from build123d import *

# Parameters (mm, degrees)
SKETCH1_R           = 13.5
BOSS_EXTRUDE1_DEPTH = 5
SKETCH2_R           = 10.65
BOSS_EXTRUDE2_DEPTH = 9.9
SKETCH5_R           = 6.1
CUT_EXTRUDE1_DEPTH  = 10


with BuildPart() as part:
    # Sketch1 → Boss-Extrude1 (new body)
    with BuildSketch(Plane.XY):
        Circle(SKETCH1_R)
    extrude(amount=BOSS_EXTRUDE1_DEPTH)

    # Sketch2 → Boss-Extrude2 (add)
    with BuildSketch(Plane.XY.offset(5)):
        with Locations(Location((0, 0, 0), (0, 0, 180))):
            Circle(SKETCH2_R)
    extrude(amount=BOSS_EXTRUDE2_DEPTH)

    # Sketch5 → Cut-Extrude1 (cut)
    with BuildSketch(Plane.XY.offset(5)):
        Circle(SKETCH5_R)
    extrude(amount=CUT_EXTRUDE1_DEPTH, mode=Mode.SUBTRACT)


solid = part.part
For this review, take the finished solid that the model builds, in its own axes (mm). A direction names the side the tool comes from. Round coordinates to 2 decimals unless told otherwise and drop trailing zeros. Loops run counter-clockwise (first coordinate to the right, second up) from the corner with the lowest first, then second, coordinate; pieces in that order, holes last. Notation, with made-up numbers: (81.5, 8.5) - (134.5, 8.5) arc R12 cw to (134.5, 29.5) - close; hole circle Ø10 at (89, 17). An arc over 180 degrees is marked (long way). Use one line per item in the form item = value.
Item 1: Tool access review of faces 5 (the flat face through (-5, 5, 14.9)), 6 (the cylindrical face through (-10.158, -3.199, 9.881)): name each direction out of +Z, -Z, +X, -X, +Y, -Y from which nothing blocks a thin tool from reaching the whole face with its end or side.
Answers:
face_5 = +Z, +X, -X, +Y, -Y
face_6 = +Z
Item 2: Consider section D-D on z = 2.75. Write out the cut boundary in (x, y), then the cut area to 3 significant figures.
Answers:
outline = circle Ø27 at (0, 0)
area = 573 mm^2
Item 3: Mouldability with a two-part tool opening along Y and no side actions: class faces 1 (the cylindrical face through (-2.93, -13.18, 2.46)), 2 (the cylindrical face through (-6.094, 0.268, 9.881)), 3 (the flat face through (0, 0, 5)), 4 (the flat face through (-10.1, -3.9, 5)) as +Y half, -Y half, draft (parallel to the pull), parting line (faces both ways), or undercut.
Answers:
face_1 = parting line
face_2 = undercut
face_3 = undercut
face_4 = draft
Item 4: Consider section A-A on z = 8. Write out the cut boundary in (x, y).
Answers:
outline = circle Ø21.3 at (0, 0); hole circle Ø12.2 at (0, 0)
Item 5: Consider section B-B on x = 0. Write out the cut boundary in (y, z), then the cut area to 3 significant figures.
Answers:
outline = (-13.5, 0) - (13.5, 0) - (13.5, 5) - (10.65, 5) - (10.65, 14.9) - (6.1, 14.9) - (6.1, 5) - (-6.1, 5) - (-6.1, 14.9) - (-10.65, 14.9) - (-10.65, 5) - (-13.5, 5) - close
area = 225 mm^2
Item 6: Clearance check with flat-ended pins moving along their axes: P1, Ø8, axis at x = 6.5, z = 11, coming from the +Y side; P2, Ø4, axis at x = -9.5, y = -8.5, coming from the +Z side; P3, Ø2, axis at x = 2, z = 2.5, coming from the +Y side. State where each tip first meets the part, or that it passes through.
Answers:
P1 = 10.35
P2 = 5
P3 = 13.46
Item 7: For line 1 (Y direction, x = 0, z = 9); line 2 (Z direction, x = -12.25, y = -3.25); line 3 (X direction, y = 1.5, z = 9.75), list the stretches that pass through material, from the lowest coordinate up.
Answers:
line_1 = -10.65 to -6.1, 6.1 to 10.65
line_2 = 0 to 5
line_3 = -10.54 to -5.91, 5.91 to 10.54
